For this review, take the finished solid that the model builds, in its own axes (mm). A direction names the side the tool comes from. Give positions to 0.01 mm unless a question says otherwise; leave off trailing zeros. Loops run counter-clockwise (first coordinate to the right, second up) from the corner with the lowest first, then second, coordinate; pieces in that order, holes last.
```python
from build123d import *

# Parameters (mm, degrees)
BOSS_EXTRUDE1_DEPTH = 5
SKETCH4_R           = 0.8
CUT_EXTRUDE3_DEPTH  = 20.474342094
SKETCH5_W           = 4
SKETCH5_H           = 3
CUT_EXTRUDE4_DEPTH  = 13
FILLET4_R           = 1
CUT_EXTRUDE5_DEPTH  = 20.474342094
FILLET6_R           = 1
CUT_EXTRUDE6_START  = -8.5
CUT_EXTRUDE6_DEPTH  = 8.002697112
SKETCH11_W          = 3
SKETCH11_H          = 5
CUT_EXTRUDE8_DEPTH  = 4
SKETCH12_R          = 0.6
CUT_EXTRUDE9_DEPTH  = 5
CUT_EXTRUDE10_REACH = 21.474
SKETCH9_R           = 0.25


# Read off the part's stored shape, not the designer's step: Cut-Extrude6
with BuildPart() as part:
    # Sketch1 → Boss-Extrude1 (new body)
    with BuildSketch(Plane.XY):
        Polygon((0, 0), (12, 0), (12, -14.5), (6.5, -14.5), (6.5, -5), (0, -5), align=None)
    extrude(amount=BOSS_EXTRUDE1_DEPTH)

    # Sketch4 → Cut-Extrude3 (cut, through all)
    with BuildSketch(Plane.XY.offset(5)):
        with Locations((1.75, -2.5)):
            Circle(SKETCH4_R)
    extrude(amount=-CUT_EXTRUDE3_DEPTH, mode=Mode.SUBTRACT)

    # Sketch5 → Cut-Extrude4 (cut)
    with BuildSketch(Plane(origin=(0, 0, 0), x_dir=(1, 0, 0), z_dir=(0, 1, 0))):
        with Locations((2, -2.5)):
            Rectangle(SKETCH5_W, SKETCH5_H)
    extrude(amount=-CUT_EXTRUDE4_DEPTH, mode=Mode.SUBTRACT)

    # Fillet4
    fillet4_edges = [part.edges().sort_by_distance(p)[0] for p in [
        (0, 0, 4.5),
        (0, -5, 4.5),
        (0, 0, 0.5),
        (0, -5, 0.5),
    ]]
    fillet(fillet4_edges, radius=FILLET4_R)

    # Sketch6 → Cut-Extrude5 (cut, through all)
    with BuildSketch(Plane.XY.offset(5)):
        Polygon((12, -13.588182425), (11, -12.588182425), (12, -11.588182425), align=None)
    extrude(amount=-CUT_EXTRUDE5_DEPTH, mode=Mode.SUBTRACT)

    # Fillet6
    fillet6_edges = [part.edges().sort_by_distance(p)[0] for p in [
        (11, -12.588182425, 2.5),
        (12, -13.588182425, 2.5),
        (12, -11.588182425, 2.5),
        (6.5, -5, 2.5),
        (6.5, -14.5, 2.5),
        (12, 0, 2.5),
    ]]
    fillet(fillet6_edges, radius=FILLET6_R - 0.0001)  # a hair under: the kernel refuses the full size

    # Cut-Extrude6 outline → Cut-Extrude6 (cut)
    with BuildSketch(Plane.XZ.offset(14.5).offset(CUT_EXTRUDE6_START)):
        with BuildLine():
            Line((6.49999436, 5.000051867), (6.499994078, -5.446e-05))
            ThreePointArc((6.499994078, -5.446e-05), (6.635532303, 2.499998696), (6.49999436, 5.000051867))
        make_face()
    extrude(amount=CUT_EXTRUDE6_DEPTH, mode=Mode.SUBTRACT)

    # Sketch11 → Cut-Extrude8 (cut, along a direction that is not the sketch's normal)
    with BuildSketch(Plane.ZY.offset(-4)):
        with Locations((2.5, -2.5)):
            Rectangle(SKETCH11_W, SKETCH11_H)
    extrude(amount=-CUT_EXTRUDE8_DEPTH, dir=(-0.8191736087025463, 0.5735456379445732, 0), mode=Mode.SUBTRACT)

    # Sketch12 → Cut-Extrude9 (cut, along a direction that is not the sketch's normal)
    with BuildSketch(Plane.ZY.offset(-6.5)):
        with Locations((3.671694189, -8.375443102)):
            Circle(SKETCH12_R)
        with Locations((3.671694189, -10.194652501)):
            Circle(SKETCH12_R)
        with Locations((3.671694189, -12.168032187)):
            Circle(SKETCH12_R)
    extrude(amount=-CUT_EXTRUDE9_DEPTH, dir=(-0.8191736087025463, 0.5735456379445732, 0), mode=Mode.SUBTRACT)

    # Cut-Extrude10: up to this plane
    cut_extrude10_end = Plane(origin=(7.276694435, -7.294182552, 1), z_dir=(-0.5735456379445732, -0.8191736087025463, 0))
    # Sketch9 → Cut-Extrude10 (cut, up to the surface)
    with BuildSketch(Plane.XZ.offset(14.5), mode=Mode.PRIVATE) as cut_extrude10_sk1:
        with Locations((6.635532303, 2.5)):
            Circle(SKETCH9_R)
    cut_extrude10_tool1 = split(extrude(cut_extrude10_sk1.sketch, amount=-CUT_EXTRUDE10_REACH, mode=Mode.PRIVATE), bisect_by=cut_extrude10_end, keep=Keep.BOTH, mode=Mode.PRIVATE)
    add(cut_extrude10_tool1.solids().sort_by_distance((6.635532, -14.5, 2.5))[0], mode=Mode.SUBTRACT)


solid = part.part
```
Item 1: The part is to be moulded in two halves that separate along Z. For faces 1 (the flat face through (0, -2.5, 4.5)), 2 (the flat face through (10.596, -11, 4)), 3 (the flat face through (7, -6, 5)), say which applies: released by +Z, released by -Z, zero draft, split by the parting line, or undercut.
Answer:
face 1: zero draft
face 2: undercut
face 3: released by +Z
Item 2: Clearance check with flat-ended pins moving along their axes: pin 1 Ø0.5 at (x, z) = (3.5, 4.5) entering from -Y; pin 2 Ø2 at (x, y) = (5, -9) entering from +Z; pin 3 Ø1 at (y, z) = (-11.5, 4) entering from -X; pin 4 Ø2 at (x, y) = (1.75, -2.5) entering from -Z. State where each tip first meets the part, or that it passes through.
Answer:
pin 1: stops at y = -5
pin 2: passes through
pin 3: stops at x = 6.55
pin 4: stops at z = 0
Item 3: Take a section at D-D on x = 5. Give the boundary of the cut face in (y, z).
Answer:
outline: (-5, 0) - (0, 0) - (0, 5) - (-5, 5) - (-5, 4) - (-0.7, 4) - (-0.7, 1) - (-5, 1) - close
Item 4: Tool access review of faces 4 (the flat face through (3.3, -5, 0.5)), 5 (the cylindrical face through (6.594, -9.944, 1.108)), 6 (the flat face through (10, -14.5, 2)): name each direction out of +Z, -Z, +X, -X, +Y, -Y from which nothing blocks a thin tool from reaching the whole face with its end or side.
Answer:
face 4: +Z, -Z, -X, -Y
face 5: -X, -Y
face 6: +Z, -Z, +X, -X, -Y
Item 5: Take a section at B-B on y = -2.5. Give the boundary of the cut face in (x, z).
Answer:
outline: (0, 0) - (0.95, 0) - (0.95, 1) - (0, 1) - close; (0, 4) - (0.95, 4) - (0.95, 5) - (0, 5) - close; (2.55, 0) - (12, 0) - (12, 5) - (2.55, 5) - (2.55, 4) - (7.28, 4) - (7.28, 1) - (2.55, 1) - close
Item 6: Take a section at A-A on x = 1.75. Give the boundary of the cut face in (y, z).
Answer:
outline: (-5, 0) - (-3.3, 0) - (-3.3, 1) - (-5, 1) - close; (-5, 4) - (-3.3, 4) - (-3.3, 5) - (-5, 5) - close; (-1.7, 0) - (0, 0) - (0, 1) - (-1.7, 1) - close; (-1.7, 4) - (0, 4) - (0, 5) - (-1.7, 5) - close
Item 7: For L1, parallel to Z at x = 6.75, y = -5.25; L2, parallel to Y at x = 8.5, z = 4.1; L3, parallel to Y at x = 1.75, z = 4.6, list the stretches that pass through material, from the lowest coordinate up.
Answer:
L1: z = 0 to 1, 4 to 5
L2: y = -14.5 to -13.99, -13.15 to -12.02, -11.17 to -10.2, -9.36 to 0
L3: y = -5 to -3.3, -1.7 to 0
